For this review, take the finished solid that the model builds, in its own axes (mm). A direction names the side the tool comes from. Round coordinates to 2 decimals unless told otherwise and drop trailing zeros. Write each loop counter-clockwise with the first axis right and the second up, starting at its lowest first coordinate (ties: lowest second). Pieces come first, ordered by that corner, then holes. Notation, with made-up numbers: M 76,-1.5 L 99,-1.5 A24 cw 99,11.5 Z; hole C -30,-30.5 d10. An arc over 180 degrees is marked long. Answer in a Markdown table with one row per item.
```python
from build123d import *

# Parameters (mm, degrees)
SKETCH_1_W          = 23
SKETCH_1_H          = 5.03
SKETCH_1_W_2        = 4.5
SKETCH_1_H_2        = 1.5
SKETCH_1_H_3        = 20.4
EXTRUDE_1_DEPTH     = 6.3
SKETCH_3_R          = 1
CUT_EXTRUDE_1_DEPTH = 10


with BuildPart() as part:
    # 草图1 → 凸台-拉伸1 (new, symmetric)
    with BuildSketch(Plane.XY):
        with Locations((0, 10.95)):
            Rectangle(SKETCH_1_W, SKETCH_1_H)
        with Locations((13.75, 7.685)):
            Rectangle(SKETCH_1_W_2, SKETCH_1_H_2)
        with Locations((0, -3.265)):
            Rectangle(SKETCH_1_W, SKETCH_1_H_3)
        with Locations((-13.75, 7.685)):
            Rectangle(SKETCH_1_W_2, SKETCH_1_H_2)
        with Locations((0, 7.685)):
            Rectangle(SKETCH_1_W, SKETCH_1_H_2)
    extrude(amount=EXTRUDE_1_DEPTH, both=True)

    # 草图2 → 旋转1 (revolve)
    with BuildSketch(Plane.XY, mode=Mode.PRIVATE) as revolve_1_sk:
        Polygon((-5.955, 13.465), (-10.52, 13.465), (-10.52, 14.735), (-8.555, 14.735), (-8.555, 18.435), (-5.955, 18.435), align=None)
    revolve(revolve_1_sk.sketch.rotate(Axis((-5.955, 10.839744531, 0), (0, 1, 0)), 270), axis=Axis((-5.955, 10.839744531, 0), (0, 1, 0)))

    # 草图3 → 切除-拉伸1 (cut)
    with BuildSketch(Plane(origin=(0, 8.435, 0), x_dir=(1, 0, 0), z_dir=(0, 1, 0))):
        with Locations(Location((-14, 3.5, 0), (0, 0, 180))):
            Circle(SKETCH_3_R)
        with Locations(Location((14, 3.5, 0), (0, 0, 180))):
            Circle(SKETCH_3_R)
        with Locations(Location((14, -3.5, 0), (0, 0, 270))):
            Circle(SKETCH_3_R)
        with Locations(Location((-14, -3.5, 0), (0, 0, 270))):
            Circle(SKETCH_3_R)
    extrude(amount=-CUT_EXTRUDE_1_DEPTH, mode=Mode.SUBTRACT)


solid = part.part
```
Q1. Mouldability with a two-part tool opening along Z and no side actions: class faces 5 (the face through (-14.976, 7.696, 3.283)), 6 (the face through (0, 0, -6.3)), 7 (the face through (11.5, -3, 0)) as +Z half, -Z half, draft (parallel to the pull), parting line (faces both ways), or undercut.
Found:
| item | result |
|---|---|
| face 5 | undercut |
| face 6 | -Z half |
| face 7 | draft |
Q2. For probe 1 along X at (y, z) = (7.3, 3.5); probe 2 along Y at (x, z) = (14.5, -2.5) (3 decimals); probe 3 along Y at (x, z) = (-9.5, 1.25) (3 decimals), list the stretches that pass through material, from the lowest coordinate up.
Found:
| item | result |
|---|---|
| probe 1 | -16 to -15, -13 to 13, 15 to 16 |
| probe 2 | 6.935 to 8.435 |
| probe 3 | -13.465 to 14.735 |
Q3. Take a section at D-D (y = -5). State the section outline as (x, z) points, then the cut area to 3 significant figures.
Found:
| item | result |
|---|---|
| outline | M -11.5,-6.3 L 11.5,-6.3 L 11.5,6.3 L -11.5,6.3 Z |
| area | 290 mm² |
Q4. Take a section at C-C (z = 4). State the section outline as (x, y) points (3 decimals).
Found:
| item | result |
|---|---|
| outline | M -16,6.935 L -14.866,6.935 L -14.866,8.435 L -16,8.435 Z; M -13.134,6.935 L -11.5,6.935 L -11.5,-13.465 L 11.5,-13.465 L 11.5,6.935 L 13.134,6.935 L 13.134,8.435 L 11.5,8.435 L 11.5,13.465 L -3.755,13.465 L -3.755,14.735 L -8.155,14.735 L -8.155,13.465 L -11.5,13.465 L -11.5,8.435 L -13.134,8.435 Z; M 14.866,6.935 L 16,6.935 L 16,8.435 L 14.866,8.435 Z |
Q5. Take a section at A-A (x = -14). State the section outline as (y, z) points (3 decimals).
Found:
| item | result |
|---|---|
| outline | M 6.935,-6.3 L 8.435,-6.3 L 8.435,-4.5 L 6.935,-4.5 Z; M 6.935,-2.5 L 8.435,-2.5 L 8.435,2.5 L 6.935,2.5 Z; M 6.935,4.5 L 8.435,4.5 L 8.435,6.3 L 6.935,6.3 Z |
Q6. Insertion check: P1, Ø4, axis at y = -3, z = 2.5, coming from the -X side; P2, Ø1.6, axis at x = 14, z = -3.5, coming from the +Y side; P3, Ø4, axis at x = 1.5, z = 4, coming from the +Y side (3 decimals); P4, Ø3, axis at x = -14, z = -3.5, coming from the +Y side (3 decimals). Each pin has a flat end and moves straight along its axis. Give the tip position at first contact, or say it passes through.
Found:
| item | result |
|---|---|
| P1 | x = -11.5 |
| P2 | through |
| P3 | y = 13.465 |
| P4 | y = 8.435 |
Q7. Take a section at B-B (z = 0). State the section outline as (x, y) points (3 decimals), then the cut area to 3 significant figures.
Found:
| item | result |
|---|---|
| outline | M -16,6.935 L -11.5,6.935 L -11.5,-13.465 L 11.5,-13.465 L 11.5,6.935 L 16,6.935 L 16,8.435 L 11.5,8.435 L 11.5,13.465 L -1.39,13.465 L -1.39,14.735 L -3.355,14.735 L -3.355,18.435 L -8.555,18.435 L -8.555,14.735 L -10.52,14.735 L -10.52,13.465 L -11.5,13.465 L -11.5,8.435 L -16,8.435 Z |
| area | 664 mm² |
Q8. Machinability: for faces 1 (the face through (14, 6.935, 0)), 2 (the face through (11.5, 11, 0)), 3 (the face through (-14, 6.935, 0)), 4 (the face through (-4, 14.735, -2)), which of the approach directions +Z, -Z, +X, -X, +Y, -Y give a long, thin tool a straight path to every point of the face, cutting with its end or side? Answer none if there is none.
Found:
| item | result |
|---|---|
| face 1 | +Z, -Z, +X, -Y |
| face 2 | +Z, -Z, +X, +Y |
| face 3 | +Z, -Z, -X, -Y |
| face 4 | +Y |
